Could you check a few things on this model? Use its own coordinates, in mm. Face numbers are marked on the shaded views. Give positions to 0.01 mm unless a question says otherwise; leave off trailing zeros. Write each loop counter-clockwise with the first axis right and the second up, starting at its lowest first coordinate (ties: lowest second). Pieces come first, ordered by that corner, then holes. Notation, with made-up numbers: M 36,0.25 L 61,0.25 A14 ccw 61,8.25 Z; hole C 40.25,33.25 d8. An arc over 180 degrees is marked long. Answer as CSV lines item,"result". Start each with the question number.
from build123d import *

# Parameters (mm, degrees)
SKETCH1_W               = 38.1
SKETCH1_H               = 3.175
BOSS_EXTRUDE1_DEPTH     = 344.17
SKETCH3_R               = 3.175
CUT_EXTRUDE1_DEPTH      = 4.175
SKETCH4_R               = 3.175
CUT_EXTRUDE2_DEPTH      = 1
CUT_EXTRUDE2_DEPTH_BACK = 4.175


with BuildPart() as part:
    # Sketch1 → Boss-Extrude1 (new body)
    with BuildSketch(Plane.XY):
        with Locations((19.05, 1.5875)):
            Rectangle(SKETCH1_W, SKETCH1_H)
    extrude(amount=BOSS_EXTRUDE1_DEPTH)

    # Sketch3 → Cut-Extrude1 (cut, through all)
    with BuildSketch(Plane(origin=(0, 3.175, 0), x_dir=(1, 0, 0), z_dir=(0, 1, 0))):
        with Locations((19.05, -227.7075202)):
            Circle(SKETCH3_R)
    extrude(amount=-CUT_EXTRUDE1_DEPTH, mode=Mode.SUBTRACT)

    # Sketch4 → Cut-Extrude2 (cut, two sides)
    with BuildSketch(Plane.XZ) as cut_extrude2_sk:
        with Locations((30.1625, 336.2325)):
            Circle(SKETCH4_R)
        with Locations((7.9375, 326.7075)):
            Circle(SKETCH4_R)
        with Locations((7.9375, 17.4625)):
            Circle(SKETCH4_R)
        with Locations((30.1625, 7.9375)):
            Circle(SKETCH4_R)
    extrude(amount=CUT_EXTRUDE2_DEPTH, mode=Mode.SUBTRACT)
    extrude(cut_extrude2_sk.sketch, amount=-CUT_EXTRUDE2_DEPTH_BACK, mode=Mode.SUBTRACT)


solid = part.part
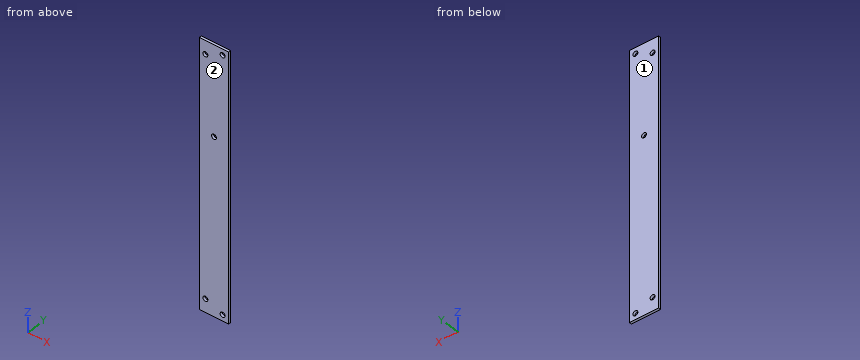
1. Please list where these lines run through material, in increasing order: line 1 (Z direction, x = 8, y = 1.15); line 2 (Z direction, x = 30, y = 0.85); line 3 (Z direction, x = 19, y = 0.8).
2. Imagine slicing it at A-A, the plane x = 19.05. Please give me the cut outline in (y, z) (3 decimals).
3. Thinking about a two-plate mould opening in Y: for the marked faces 1 and 2, which applies, pulls with the +Y half, pulls with the -Y half, needs draft (parallel to the pull), parting line crosses it, or undercut?
Solutions:
1,line 1,"0 to 14.29, 20.64 to 323.53, 329.88 to 344.17"
1,line 2,"0 to 4.77, 11.11 to 333.06, 339.4 to 344.17"
1,line 3,"0 to 224.53, 230.88 to 344.17"
2,outline,"M 0,0 L 3.175,0 L 3.175,224.533 L 0,224.533 Z; M 0,230.883 L 3.175,230.883 L 3.175,344.17 L 0,344.17 Z"
3,face 1,"pulls with the +Y half"
3,face 2,"pulls with the -Y half"
